Build history of the part. All positions in model axes, mm. Face numbers are marked on the shaded views. A direction names the side the tool comes from. Round coordinates to 2 decimals unless told otherwise and drop trailing zeros. Write each loop counter-clockwise with the first axis right and the second up, starting at its lowest first coordinate (ties: lowest second). Pieces come first, ordered by that corner, then holes.
1) Saw through at A-A (y = 25.5). Write the cut outline in (x, z), plus the area to 3 significant figures.
2) Wall check: probe 1 along Z at (x, y) = (1, 8.5); probe 2 along Y at (x, z) = (5, 7.25); probe 3 along Z at (x, y) = (7.25, -16). Give the ranges that are in metal, low to high.
3) Flat gauge pin, fed straight in: pin 1 (10 mm diameter, centred on x = 2.5, y = 24.5, fed in from +Z). Where does the tip first touch, or does it go through?
4) Which spindle directions (+Z, -Z, +X, -X, +Y, -Y) get a long thin tool onto all of the face, cutting with end or side? Do the marked faces 1 and 2. Say none if no direction does.
from build123d import *

# Parameters (mm, degrees)
F0_W        = 25.9
F0_H        = 57
F1_DEPTH    = 8.2
F2_W        = 25.9
F2_H        = 12.2
F3_DEPTH    = 4
F4_T1_DEPTH = 65.9
F5_R        = 5


# Not quite as in the source:
# - a fillet or chamfer that OpenCascade refuses, or shapes differently, is made with other operations: its cross-section is extruded or revolved along the edge and cut away or added


with BuildPart() as f1:
    # F0 (on Top) → F1 (new body)
    with BuildSketch(Plane.XY):
        with Locations((8.0425532069, 7.3918554072)):
            Rectangle(F0_W, F0_H)
    extrude(amount=F1_DEPTH)

    # F2 (on face) → F3 (join)
    with BuildSketch(Plane.XY.offset(8.2)):
        with Locations((8.0425532069, -15.0081445928)):
            Rectangle(F2_W, F2_H)
    extrude(amount=F3_DEPTH)

    # F4: fillet of radius 10 on 1 edges, made by hand

    # F4_s2 → F4_t1 (cut)
    with BuildSketch(Plane.YZ.offset(-24.9074467931)):
        with BuildLine():
            ThreePointArc((-8.9081445928, 8.2), (-12.4360086378, 11.14427191), (-16.9081445928, 12.2))
            Line((-16.9081445928, 12.2), (-8.9081445928, 12.2))
            Line((-8.9081445928, 12.2), (-8.9081445928, 8.2))
        make_face()
    extrude(amount=F4_T1_DEPTH, mode=Mode.SUBTRACT)

    # F5
    f5_edges = [f1.edges().sort_by_distance(p)[0] for p in [
        (8.042553, -21.108145, 12.2),
    ]]
    fillet(f5_edges, radius=F5_R)


solid = f1.part
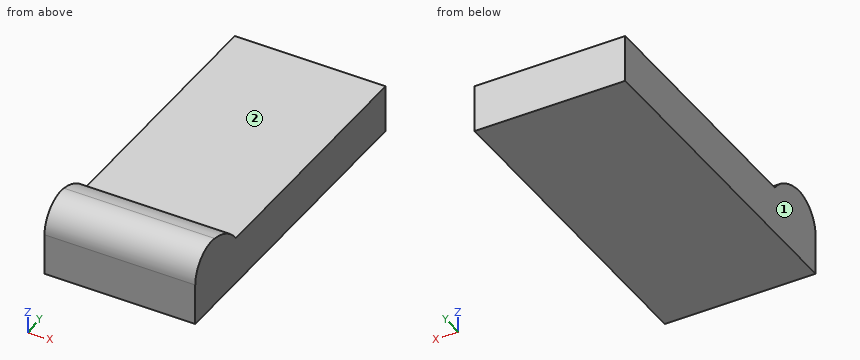
Evaluation:
1. outline: (-4.91, 0) - (20.99, 0) - (20.99, 8.2) - (-4.91, 8.2) - close
1. area: 212 mm2
2. probe 1: z = 0 to 8.2
2. probe 2: y = -21.11 to 35.89
2. probe 3: z = 0 to 12.13
3. pin 1: stops at z = 8.2
4. face 1: +Z, -Z, -X, +Y, -Y
4. face 2: +Z, +X, -X, +Y
